Design review of the part built by this model. Coordinates are the model's own, in mm. A direction names the side the tool comes from. Give positions to 0.01 mm unless a question says otherwise; leave off trailing zeros. Write each loop counter-clockwise with the first axis right and the second up, starting at its lowest first coordinate (ties: lowest second). Pieces come first, ordered by that corner, then holes. Notation, with made-up numbers: (31.5, -29.5) -> (82.5, -29.5) arc R24 ccw to (82.5, 2.5) -> close; hole circle Ø5 at (48.5, 5). An arc over 180 degrees is marked (long way). Use CSV: the item, a comma, the result in double quotes.
```python
from build123d import *

# Parameters (mm, degrees)
F0_W     = 101.6
F0_H     = 147
F0_R     = 3
F1_DEPTH = 1.5
F2_R     = 1.6
F3_DEPTH = 25
F4_DEPTH = 5
F5_R     = 1.5
F6_DEPTH = 3
F7_W     = 101.6
F7_H     = 44.8
F8_DEPTH = 25
F9_R     = 5


# Not quite as in the source:
# - a feature names something its author has since deleted; it is built from what else it names


with BuildPart() as f1:
    # F0 (on Top) → F1 (new body)
    with BuildSketch(Plane.XY):
        with Locations((-19.733554095, 37.0265730321)):
            Rectangle(F0_W, F0_H)
        with Locations((-67.358554095, 24.7965730321)):
            Circle(F0_R, mode=Mode.SUBTRACT)
        with Locations((27.891445905, 24.7965730321)):
            Circle(F0_R, mode=Mode.SUBTRACT)
        with Locations((-67.358554095, 69.2465730321)):
            Circle(F0_R, mode=Mode.SUBTRACT)
        with Locations((27.891445905, 69.2465730321)):
            Circle(F0_R, mode=Mode.SUBTRACT)
    extrude(amount=F1_DEPTH)

    # F2 (on face) → F3 (cut)
    with BuildSketch(Plane.XY.offset(1.5)):
        with Locations((-67.358554095, 96.5265730321)):
            Circle(F2_R)
        with Locations((-5.758554095, 96.5265730321)):
            Circle(F2_R)
        with Locations((-67.358554095, 19.9265730321)):
            Circle(F2_R)
        with Locations((-5.758554095, 19.9265730321)):
            Circle(F2_R)
    extrude(amount=-F3_DEPTH, mode=Mode.SUBTRACT)

    # F0 (on Top) → F4 (join)
    with BuildSketch(Plane.XY):
        with Locations((-67.358554095, 69.2465730321)):
            Circle(F0_R)
        with Locations((-67.358554095, 24.7965730321)):
            Circle(F0_R)
        with Locations((27.891445905, 69.2465730321)):
            Circle(F0_R)
        with Locations((27.891445905, 24.7965730321)):
            Circle(F0_R)
    extrude(amount=F4_DEPTH)

    # F5 (on face) → F6 (cut)
    with BuildSketch(Plane.XY.offset(5)):
        with Locations((-67.358554095, 69.2465730321)):
            Circle(F5_R)
        with Locations((-67.358554095, 24.7965730321)):
            Circle(F5_R)
        with Locations((27.891445905, 69.2465730321)):
            Circle(F5_R)
        with Locations((27.891445905, 24.7965730321)):
            Circle(F5_R)
    extrude(amount=-F6_DEPTH, mode=Mode.SUBTRACT)

    # F7 (on face) → F8 (cut)
    with BuildSketch(Plane.XY.offset(1.5)):
        with Locations((-19.733554095, -14.0734269679)):
            Rectangle(F7_W, F7_H)
        Polygon((-70.533554095, 8.3265730321), (-108.6030122084, 8.3265730321), (-108.6030122084, -69.3553299345), (74.6913593453, -69.3553299345), (74.6913593453, 8.3265730321), (31.066445905, 8.3265730321), (31.066445905, -36.4734269679), (-70.533554095, -36.4734269679), align=None)
        Polygon((-108.166599336, 100.5265730321), (-70.533554095, 100.5265730321), (-70.533554095, 110.5265730321), (31.066445905, 110.5265730321), (31.066445905, 100.5265730321), (58.5440034669, 100.5265730321), (58.5440034669, 119.7288488672), (-108.166599336, 119.7288488672), align=None)
    extrude(amount=-F8_DEPTH, mode=Mode.SUBTRACT)

    # F9
    f9_edges = [f1.edges().sort_by_distance(p)[0] for p in [
        (-70.533554, 8.326573, 0.75),
        (-70.533554, 110.526573, 0.75),
        (31.066446, 8.326573, 0.75),
        (31.066446, 110.526573, 0.75),
    ]]
    fillet(f9_edges, radius=F9_R)


solid = f1.part
```
(1) For line 1 along X through (y, z) = (20, 0.75); line 2 along Z through (x, y) = (-53, 43); line 3 along X through (y, z) = (68.5, 1.7), list the stretches that pass through material, from the lowest coordinate up. Write a range as [from, to].
Established:
line 1,"x = [-70.53, -68.96], [-65.76, -7.36], [-4.16, 31.07]"
line 2,"z = [0, 1.5]"
line 3,"x = [-70.26, -64.45], [24.99, 30.8]"
(2) Tool access review of faces 1 (the face through (-67.567, 21.513, 0.76)), 2 (the face through (25.68, 26.824, 3.226)): name each direction out of +Z, -Z, +X, -X, +Y, -Y from which nothing blocks a thin tool from reaching the whole face with its end or side.
Established:
face 1,"+Z, -Z"
face 2,"+Z"
(3) Clearance check with flat-ended pins moving along their axes: pin 1 (4 mm diameter, centred on x = -30, y = 71, fed in from +Z); pin 2 (2.5 mm diameter, centred on x = -67.36, y = 69.25, fed in from +Z); pin 3 (2 mm diameter, centred on y = 39.5, z = 3, fed in from -X). State where each tip first meets the part, or that it passes through.
Established:
pin 1,"stops at z = 1.5"
pin 2,"stops at z = 2"
pin 3,"passes through"
(4) Take a section at A-A (z = 3.6). Write out the cut boundary in (x, y).
Established:
outline,"circle Ø6 at (-67.36, 24.8); circle Ø6 at (-67.36, 69.25); circle Ø6 at (27.89, 24.8); circle Ø6 at (27.89, 69.25); hole circle Ø3 at (-67.36, 24.8); hole circle Ø3 at (-67.36, 69.25); hole circle Ø3 at (27.89, 24.8); hole circle Ø3 at (27.89, 69.25)"
(5) Take a section at C-C (y = 104). Write out the cut boundary in (x, z).
Established:
outline,"(-70.53, 0) -> (31.07, 0) -> (31.07, 1.5) -> (-70.53, 1.5) -> close"
(6) Take a section at B-B (x = 16). Write out the cut boundary in (y, z), then the cut area to 3 significant figures.
Established:
outline,"(8.33, 0) -> (110.53, 0) -> (110.53, 1.5) -> (8.33, 1.5) -> close"
area,"153 mm2"
(7) Mouldability with a two-part tool opening along X and no side actions: class faces 3 (the face through (-69, 24, 5)), 4 (the face through (-66.666, 23.466, 3.521)), 5 (the face through (-69.03, 9.75, 0.74)), 6 (the face through (-65.974, 66.585, 3.226)) as +X half, -X half, draft (parallel to the pull), parting line (faces both ways), or undercut.
Established:
face 3,"draft"
face 4,"undercut"
face 5,"-X half"
face 6,"undercut"
